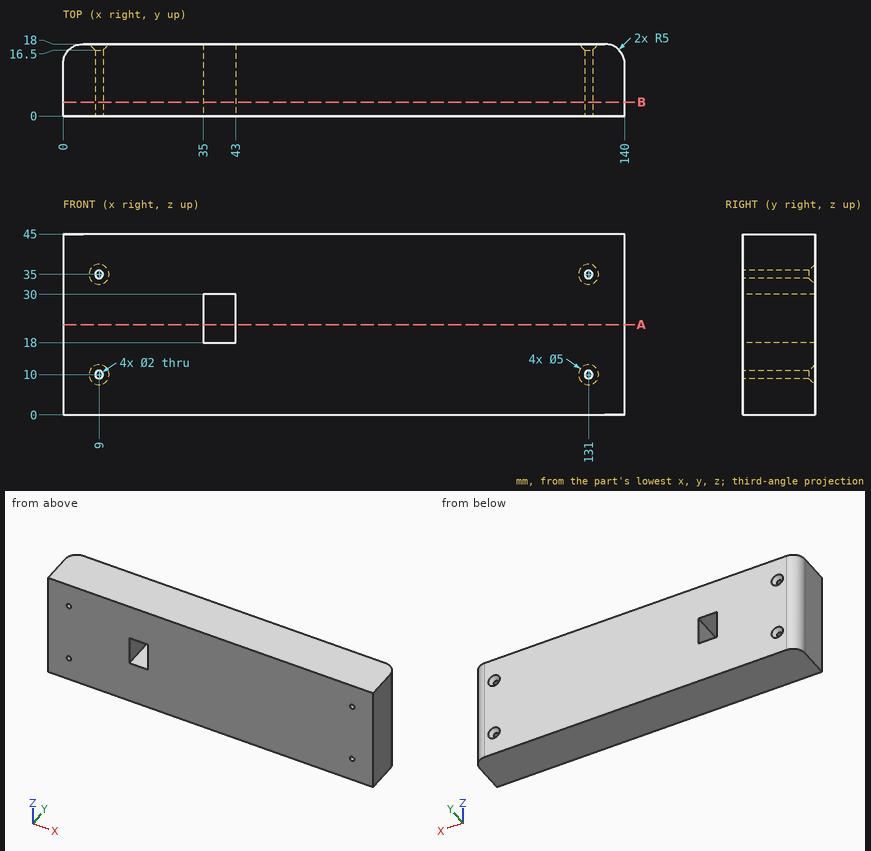
Study the drawing (mm; zero at the part's minimum x, y, z) and answer. Give positions to 0.01 mm unless a question says otherwise; leave off trailing zeros. Order: outer loops, then holes, each group sorted by start corner. A loop starts at its lowest first (then second) coordinate and runs counter-clockwise, first axis right, second up. Notation, with made-up numbers: (10.25, 9) - (49.25, 9) arc R12 ccw to (49.25, 30) - close; hole circle Ø4 at (-4, -2.5). An arc over 180 degrees is marked (long way). Use one line per item in the form item = value. Start each with the question number.
(1) Consider line 1 (Z direction, x = 131, y = 12.5); line 2 (X direction, y = 4.75, z = 35); line 3 (X direction, y = 13.75, z = 28.5). Determine where each line is inside the solid, lowest interval first. Write a range as from..to.
(2) A cutting plane is placed at A-A, the plane z = 22.5. Write down the section's boundary in (x, y), then the cut area to 3 significant figures.
(3) A cutting plane is placed at B-B, the plane y = 3.5. Write down the section's boundary in (x, z).
Ans:
q1.line_1 = 0..9, 11..34, 36..45
q1.line_2 = 0..8, 10..130, 132..140
q1.line_3 = 0.06..35, 43..139.94
q2.outline = (0, 0) - (35, 0) - (35, 18) - (5, 18) arc R5 ccw to (0, 13) - close; (43, 0) - (140, 0) - (140, 13) arc R5 ccw to (135, 18) - (43, 18) - close
q2.area = 2,370 mm^2
q3.outline = (0, 0) - (140, 0) - (140, 45) - (0, 45) - close; hole circle Ø2 at (9, 10); hole circle Ø2 at (9, 35); hole (35, 18) - (43, 18) - (43, 30) - (35, 30) - close; hole circle Ø2 at (131, 10); hole circle Ø2 at (131, 35)
